Build history of the part. All positions in model axes, mm. A direction names the side the tool comes from. Round coordinates to 2 decimals unless told otherwise and drop trailing zeros. Write each loop counter-clockwise with the first axis right and the second up, starting at its lowest first coordinate (ties: lowest second). Pieces come first, ordered by that corner, then holes. Notation, with made-up numbers: M 45,68 L 71,68 A23 cw 71,79 Z; hole C -7.75,29.25 d11. An arc over 180 degrees is marked long. Write item = value, one per line. Start each with the question number.
Q1. Drop flat-ended pins along their axis: P1, Ø4, axis at x = -7.5, z = -14, coming from the -Y side; P2, Ø4, axis at x = 30, z = -21, coming from the +Y side; P3, Ø3, axis at y = 6, z = -16, coming from the -X side. Give the stop position or say it passes through.
Q2. Probe L1, parallel to Y at x = 28, z = -16.5; L2, parallel to X at y = 10, z = -3; L3, parallel to X at y = 5.5, z = -15. List the from-to ranges inside material, lowest first.
Q3. Band-saw the part on C-C on x = 16.5. Write the cut outline in (y, z), plus the area to 3 significant figures.
Q4. Band-saw the part on A-A on y = 8. Write the cut outline in (x, z), plus the area to 3 significant figures.
Q5. Pull direction Y, two halves, no side cores. Call faces 1 (the flat face through (116.25, 12.99, -12.22)), 2 (the cylindrical face through (115, -1, -12)), 3 (the flat face through (109.245, 29.107, -12.221)), 4 (the cylindrical face through (116.85, 25.3, -12.22)): released by +Y, released by -Y, zero draft, split by the parting line, or undercut.
Q6. Band-saw the part on D-D on y = 25. Write the cut outline in (x, z).
Q7. Band-saw the part on B-B on z = -10.5. Write the cut outline in (x, y).
Q8. Tool access for faces 5 (the cylindrical face through (114.011, 0.773, -12.221)), 6 (the flat face through (108.835, 27.142, -12.221)), 7 (the flat face through (-11.46, 9.28, -12.57)): list every direction of +Z, -Z, +X, -X, +Y, -Y with a clear straight run to the whole face (end or side of a thin tool).
```python
from build123d import *

# Parameters (mm, degrees)
SKETCH_1_W             = 112
SKETCH_1_H             = 24.788135593
SM_BASE_FLANGE_1_DEPTH = 2
SM_EDGE_FLANGE_1_DEPTH = 24.788135593
SM_EDGE_FLANGE_2_DEPTH = 24.788135593
SM_EDGE_FLANGE_3_DEPTH = 24.788135593


# Sheet-metal steps are written as plain solids
with BuildPart() as part:
    # Sketch 1 → Базовая кромка1 (new body)
    with BuildSketch(Plane(origin=(0, 0, 0), x_dir=(1, 0, 0), z_dir=(0, 1, 0))):
        with Locations((56, 12.394067796)):
            Rectangle(SKETCH_1_W, SKETCH_1_H)
    extrude(amount=-SM_BASE_FLANGE_1_DEPTH)

    # Ребро-кромка1 section (across the edge) → Ребро-кромка1 (add)
    with BuildSketch(Plane(origin=(114.654175794, 0, 0), x_dir=(-0.9925461516413217, 0.12186934340515113, 0), z_dir=(0, 0, -1))):
        with BuildLine():
            Line((-2, 2.654175794), (-2, 23.230549471))
            Line((-2, 23.230549471), (0, 23.230549471))
            Line((0, 23.230549471), (0, 2.654175794))
            ThreePointArc((0, 2.654175794), (0.753132838, 0.666315649), (2.63439197, -0.323462661))
            Line((2.63439197, -0.323462661), (2.390653283, -2.308554965))
            ThreePointArc((2.390653283, -2.308554965), (-0.744778604, -0.658924447), (-2, 2.654175794))
        make_face()
    extrude(amount=SM_EDGE_FLANGE_1_DEPTH)

    # Ребро-кромка2 section (across the edge) → Ребро-кромка2 (add)
    with BuildSketch(Plane(origin=(117.850875635, 26.035030933, 0), x_dir=(-0.12186934340515466, -0.9925461516413212, 0), z_dir=(0, 0, -1))):
        with BuildLine():
            Line((-2, 3), (-2, 15))
            Line((-2, 15), (0, 15))
            Line((0, 15), (0, 3))
            ThreePointArc((0, 3), (0.878679656, 0.878679656), (3, 0))
            Line((3, 0), (3, -2))
            ThreePointArc((3, -2), (-0.535533906, -0.535533906), (-2, 3))
        make_face()
    extrude(amount=SM_EDGE_FLANGE_2_DEPTH)

    # Ребро-кромка3 section (across the edge) → Ребро-кромка3 (add)
    with BuildSketch(Plane(origin=(-1.151592105, 0, -24.788135593), x_dir=(0.6691306063588548, 0.7431448254773974, 0), z_dir=(0, 0, 1))):
        with BuildLine():
            Line((-2, 1.151592105), (-2, 26.23227193))
            Line((-2, 26.23227193), (0, 26.23227193))
            Line((0, 26.23227193), (0, 1.151592105))
            ThreePointArc((0, 1.151592105), (0.199258721, 0.076488256), (0.770565524, -0.855799714))
            Line((0.770565524, -0.855799714), (-0.715724127, -2.194060927))
            ThreePointArc((-0.715724127, -2.194060927), (-1.667902132, -0.640247643), (-2, 1.151592105))
        make_face()
    extrude(amount=SM_EDGE_FLANGE_3_DEPTH)


solid = part.part
```
Conclusion:
q1.P1 = 1.22
q1.P2 = 0
q1.P3 = -12.47
q2.L1 = -2 to 0
q2.L2 = -15.25 to -12.26, 115.88 to 117.9
q2.L3 = -10.25 to -7.26, 115.33 to 117.34
q3.outline = M -2,-24.79 L 0,-24.79 L 0,0 L -2,0 Z
q3.area = 49.6 mm^2
q4.outline = M -13.03,-24.79 L -10.04,-24.79 L -10.04,0 L -13.03,0 Z; M 115.64,-24.79 L 117.65,-24.79 L 117.65,0 L 115.64,0 Z
q4.area = 124 mm^2
q5.face_1 = undercut
q5.face_2 = released by -Y
q5.face_3 = released by +Y
q5.face_4 = undercut
q6.outline = M 117.06,-24.79 L 119.25,-24.79 L 119.25,0 L 117.06,0 Z
q7.outline = M -21.98,16.07 L -3.35,-0.72 A5 ccw 0,-2 L 112,-2 A5 ccw 116.96,2.39 L 119.47,22.81 A5 ccw 115.12,28.39 L 103.21,29.85 L 102.96,27.86 L 114.87,26.4 A3 cw 117.49,23.06 L 114.98,2.63 A3 cw 112,0 L 0,0 A3 cw -2.01,0.77 L -20.65,17.55 Z
q8.face_5 = +Z, -Z
q8.face_6 = +Z, -Z, -X
q8.face_7 = +Z, -Z, +Y
